Job drawing, mm, ordinate dimensions from the low corner. One solid piece. Round coordinates to 2 decimals unless told otherwise and drop trailing zeros. Loops run counter-clockwise (first coordinate to the right, second up) from the corner with the lowest first, then second, coordinate; pieces in that order, holes last. Notation, with made-up numbers: M 11.25,-1 L 61.25,-1 A21 cw 61.25,38 Z; hole C 87,-32 d9. An arc over 180 degrees is marked long. Use a Markdown table: item, result. Add a question column.
(1) Band-saw the part on D-D, the plane z = 7.75. Write the cut outline in (x, y) (3 decimals), and give its area (3 significant figures).
(2) Band-saw the part on C-C, the plane y = 79. Write the cut outline in (x, z) (3 decimals).
(3) Band-saw the part on A-A, the plane x = 80. Write the cut outline in (y, z), and give its area (3 significant figures).
(4) Band-saw the part on B-B, the plane y = 51. Write the cut outline in (x, z) (3 decimals).
(5) Wall check: L1, parallel to X at y = 78.5, z = 2.25 (3 decimals); L2, parallel to X at y = 47.5, z = 9.75 (3 decimals); L3, parallel to Y at x = 101.5, z = 8.5. Give the ranges that are in metal, low to high.
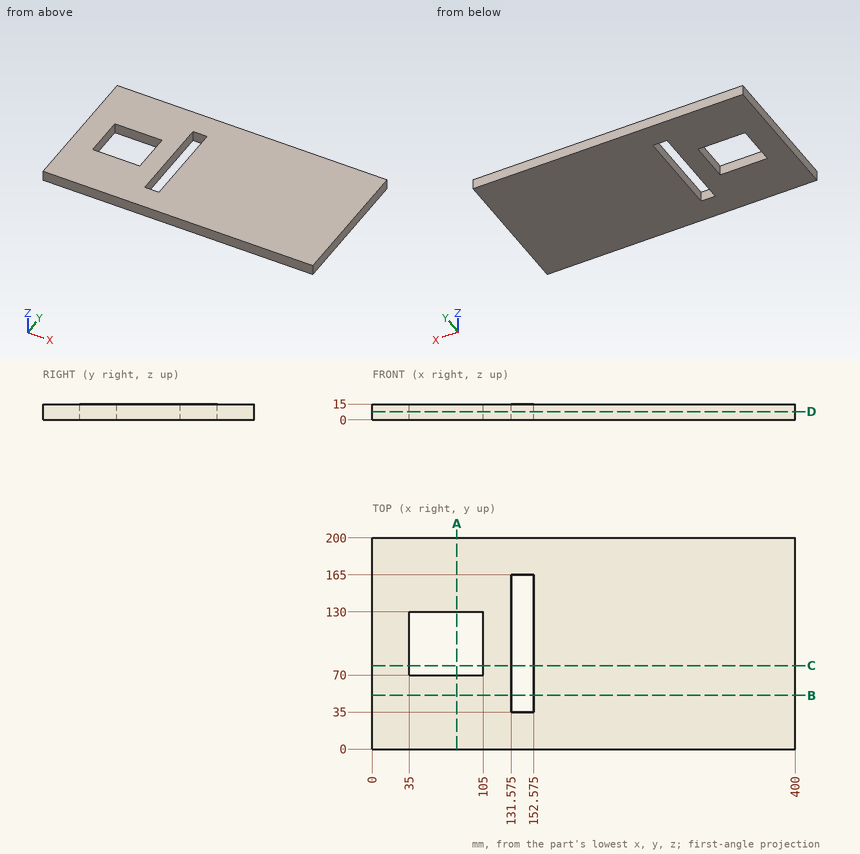
Return value:
| question | item | result |
|---|---|---|
| 1 | outline | M 0,0 L 400,0 L 400,200 L 0,200 Z; hole M 35,70 L 105,70 L 105,130 L 35,130 Z; hole M 131.575,35 L 152.575,35 L 152.575,165 L 131.575,165 Z |
| 1 | area | 73,100 mm^2 |
| 2 | outline | M 0,0 L 35,0 L 35,15 L 0,15 Z; M 105,0 L 131.575,0 L 131.575,15 L 105,15 Z; M 152.575,0 L 400,0 L 400,15 L 152.575,15 Z |
| 3 | outline | M 0,0 L 70,0 L 70,15 L 0,15 Z; M 130,0 L 200,0 L 200,15 L 130,15 Z |
| 3 | area | 2,100 mm^2 |
| 4 | outline | M 0,0 L 131.575,0 L 131.575,15 L 0,15 Z; M 152.575,0 L 400,0 L 400,15 L 152.575,15 Z |
| 5 | L1 | 0 to 35, 105 to 131.575, 152.575 to 400 |
| 5 | L2 | 0 to 131.575, 152.575 to 400 |
| 5 | L3 | 0 to 70, 130 to 200 |
